Model file for the job. Use its own axes, mm. A direction names the side the tool comes from. Coordinates: 2 decimals unless noted, no trailing zeros. Order: outer loops, then holes, each group sorted by start corner. A loop starts at its lowest first (then second) coordinate and runs counter-clockwise, first axis right, second up. Notation, with made-up numbers: (15.5, -33.5) -> (24.5, -33.5) arc R22 ccw to (24.5, 0.5) -> close; hole circle Ø2 at (58, -31). An arc over 180 degrees is marked (long way). Return JSON: item names as keys, results as strings. Group by question number.
1) Probe line 1 (Z direction, x = 2.15, y = 30); line 2 (Z direction, x = 2.55, y = 5.5); line 3 (Z direction, x = 2.35, y = -5.5). List the from-to ranges inside material, lowest first.
2) Cut at B-B (z = 117). Write the cut outline in (x, y).
3) Cut at A-A (y = -22.5). Write the cut outline in (x, z).
4) Cut at D-D (y = -40). Write the cut outline in (x, z), and give its area (3 significant figures).
5) Pull direction Y, two halves, no side cores. Call faces 1 (the cylindrical face through (2.81, 2.419, 106.266)), 2 (the flat face through (3, 38, 140.35)), 3 (the flat face through (3, 50.8, 2)): +Y half, -Y half, draft (parallel to the pull), parting line (faces both ways), or undercut.
6) Flat gauge pins, fed straight in: pin 1 (3 mm diameter, centred on x = 4, z = -143.5, fed in from -Y); pin 2 (1.7 mm diameter, centred on x = 4, y = 37.5, fed in from +Z); pin 3 (3 mm diameter, centred on x = 3.5, y = 39.5, fed in from -Z). Where does each tip first touch, or does it go through?
7) Cut at C-C (x = 3.55). Write the cut outline in (y, z), and give its area (3 significant figures).
8) Which spindle directions (+Z, -Z, +X, -X, +Y, -Y) get a long thin tool onto all of the face, cutting with end or side? Do faces 4 (the flat face through (3, -25.05, 143)), 5 (the flat face through (3, 25.75, -143)), 6 (the flat face through (5.7, 1, -2)), 7 (the flat face through (3, 25.75, 143)), 8 (the flat face through (3, -38, -140.35)). Say none if no direction does.
from build123d import *

# Parameters (mm, degrees)
SKETCH1_R           = 4.15
SKETCH1_R_2         = 10.345352818
SKETCH1_R_3         = 14.85
BOSS_EXTRUDE1_DEPTH = 5.7


with BuildPart() as part:
    # Sketch1 → Boss-Extrude1 (new body)
    with BuildSketch(Plane(origin=(0, 0, 0), x_dir=(0, 0, -1), z_dir=(1, 0, 0))):
        Polygon((-140.35, 50.8), (140.35, 50.8), (140.35, 25.75), (146.05, 25.75), (146.05, -25.05), (140.35, -25.05), (140.35, -50.8), (-140.35, -50.8), (-140.35, -25.05), (-146.05, -25.05), (-146.05, 25.75), (-140.35, 25.75), align=None)
        with Locations((131.642431314, 25.75)):
            Circle(SKETCH1_R, mode=Mode.SUBTRACT)
        with Locations((-116.133665793, -0.68799565)):
            Circle(SKETCH1_R_2, mode=Mode.SUBTRACT)
        with Locations((-115.858467533, -30.959804269)):
            Circle(SKETCH1_R_3, mode=Mode.SUBTRACT)
    extrude(amount=BOSS_EXTRUDE1_DEPTH)


solid = part.part
Answers below:
{
 "1": {"line 1": "z = -140.35 to 140.35", "line 2": "z = -146.05 to 107.84, 124.42 to 146.05", "line 3": "z = -146.05 to 106.98, 125.29 to 146.05"},
 "2": {"outline": "(0, -50.8) -> (5.7, -50.8) -> (5.7, -45.77) -> (0, -45.77) -> close; (0, -16.15) -> (5.7, -16.15) -> (5.7, -11) -> (0, -11) -> close; (0, 9.62) -> (5.7, 9.62) -> (5.7, 50.8) -> (0, 50.8) -> close"},
 "3": {"outline": "(0, -146.05) -> (5.7, -146.05) -> (5.7, 103.65) -> (0, 103.65) -> close; (0, 128.06) -> (5.7, 128.06) -> (5.7, 146.05) -> (0, 146.05) -> close"},
 "4": {"outline": "(0, -140.35) -> (5.7, -140.35) -> (5.7, 104.08) -> (0, 104.08) -> close; (0, 127.64) -> (5.7, 127.64) -> (5.7, 140.35) -> (0, 140.35) -> close", "area": "1,470 mm^2"},
 "5": {"face 1": "undercut", "face 2": "draft", "face 3": "+Y half"},
 "6": {"pin 1": "stops at y = -25.05", "pin 2": "stops at z = 140.35", "pin 3": "stops at z = -140.35"},
 "7": {"outline": "(-50.8, -140.35) -> (-25.05, -140.35) -> (-25.05, -146.05) -> (25.75, -146.05) -> (25.75, -140.35) -> (50.8, -140.35) -> (50.8, 140.35) -> (25.75, 140.35) -> (25.75, 146.05) -> (-25.05, 146.05) -> (-25.05, 140.35) -> (-50.8, 140.35) -> close; hole circle Ø29.7 at (-30.96, 115.86); hole circle Ø20.69 at (-0.69, 116.13); hole circle Ø8.3 at (25.75, -131.64)", "area": "28,000 mm^2"},
 "8": {"face 4": "+Z, +X, -X, -Y", "face 5": "-Z, +X, -X, +Y", "face 6": "+Z, -Z, +X, +Y, -Y", "face 7": "+Z, +X, -X, +Y", "face 8": "-Z, +X, -X, -Y"}
}
